Could you check a few things on this model? Use its own coordinates, in mm. A direction names the side the tool comes from. Give positions to 0.01 mm unless a question says otherwise; leave off trailing zeros. Order: outer loops, then holes, each group sorted by start corner. A loop starts at its lowest first (then second) coordinate and runs counter-clockwise, first axis right, second up. Notation, with made-up numbers: (6, 74) -> (33, 74) arc R27 ccw to (33, 100) -> close; hole circle Ø2 at (-30, 38.25). An arc over 180 degrees is marked (long way). One line per item, written item: value.
```python
from build123d import *

# Parameters (mm, degrees)
F0_W     = 20
F0_H     = 40
F0_R     = 2.75
F1_DEPTH = 4
F2_W     = 20
F2_H     = 10
F3_DEPTH = 15
F4_W     = 8.5
F4_H     = 4.5
F5_DEPTH = 30
F6_R     = 2.5
F7_DEPTH = 20
F9_DEPTH = 3


# Not quite as in the source:
# - a pattern or mirror of a feature is missing from the dataset's text; its kind, count and spacing are read off the source's solid


with BuildPart() as f1:
    # F0 (on Front) → F1 (new body)
    with BuildSketch(Plane.XZ):
        Rectangle(F0_W, F0_H)
        with Locations((0, -10)):
            Circle(F0_R, mode=Mode.SUBTRACT)
        with Locations((0, 10)):
            Circle(F0_R, mode=Mode.SUBTRACT)
    extrude(amount=F1_DEPTH)

    # F2 (on face) → F3 (join)
    with BuildSketch(Plane(origin=(0, 0, 0), x_dir=(-1, 0, 0), z_dir=(0, 1, 0))):
        with Locations((0, 20)):
            Rectangle(F2_W, F2_H)
    extrude(amount=-F3_DEPTH)

    # F4 (on face) → F5 (cut)
    with BuildSketch(Plane.XZ.offset(15)):
        with Locations((0, 20)):
            Rectangle(F4_W, F4_H)
    extrude(amount=-F5_DEPTH, mode=Mode.SUBTRACT)

    # F6 (on face) → F7 (cut)
    with BuildSketch(Plane.XY.offset(25)):
        with Locations((0, -10)):
            Circle(F6_R)
    extrude(amount=-F7_DEPTH, mode=Mode.SUBTRACT)

    # F8 (on face) → F9 (join)
    with BuildSketch(Plane(origin=(-10, 0, 0), x_dir=(0, -1, 0), z_dir=(-1, 0, 0))):
        Polygon((4, -20), (15, 15), (4, 15), align=None)
    f9 = extrude(amount=-F9_DEPTH)

    # F9_copies: F9 across plane
    add(f9.mirror(Plane(origin=(0, 0, 0), x_dir=(0, 0, 1), z_dir=(1, 0, 0))))


solid = f1.part
```
1) For P1, Ø8, axis at x = 0, y = -10, coming from the -Z side; P2, Ø9, axis at y = -10.5, z = -1.5, coming from the +X side; P3, Ø4, axis at x = 2, z = -9, coming from the -Y side, each with a flat end and sliding along its axis, tell me the tip position at first contact or that it passes through.
Answer below:
P1: stops at z = 15
P2: stops at x = 10
P3: stops at y = -4
2) Suppose I cut it at D-D, the plane x = 3.5. Write out the boundary of the cut face in (y, z).
Answer below:
outline: (-15, 15) -> (-4, 15) -> (-4, -20) -> (0, -20) -> (0, 17.75) -> (-15, 17.75) -> close; (-15, 22.25) -> (0, 22.25) -> (0, 25) -> (-15, 25) -> close
3) Suppose I cut it at C-C, the plane y = -9.25. Write out the boundary of the cut face in (x, z).
Answer below:
outline: (-10, -3.3) -> (-7, -3.3) -> (-7, 15) -> (-2.38, 15) -> (-2.38, 17.75) -> (-4.25, 17.75) -> (-4.25, 22.25) -> (-2.38, 22.25) -> (-2.38, 25) -> (-10, 25) -> close; (2.38, 15) -> (7, 15) -> (7, -3.3) -> (10, -3.3) -> (10, 25) -> (2.38, 25) -> (2.38, 22.25) -> (4.25, 22.25) -> (4.25, 17.75) -> (2.38, 17.75) -> close
4) For faces 5 (the flat face through (8.521, -9.423, -2.745)), 6 (the flat face through (4.25, -8, 20)), 7 (the flat face through (0, -7, 15)), which set-ups out of +Z, -Z, +X, -X, +Y, -Y let a thin tool reach every point of the face, with its end or its side?
Answer below:
face 5: -Z, +X, -X, -Y
face 6: +Y, -Y
face 7: -Z, -Y
5) We'd pull the mould along Z, two halves only. Please class faces 1 (the flat face through (7, -8, 2)), 2 (the flat face through (0, -6, 17.75)), 3 (the flat face through (-4.25, -8, 20)), 4 (the flat face through (-8.521, -9.423, -2.745)): +Z half, -Z half, draft (parallel to the pull), parting line (faces both ways), or undercut.
Answer below:
face 1: draft
face 2: undercut
face 3: undercut
face 4: -Z half
6) If I drill on line 1 along Z through (x, y) = (0, -0.75); line 2 along X through (y, z) = (-6.5, 3.5); line 3 along Y through (x, z) = (0, 16.15), over which ranges is the centre line in solid material (lowest first)?
Answer below:
line 1: z = -20 to -12.75, -7.25 to 7.25, 12.75 to 17.75, 22.25 to 25
line 2: x = -10 to -7, 7 to 10
line 3: y = -15 to -12.5, -7.5 to 0
7) Suppose I cut it at B-B, the plane x = 0. Write out the boundary of the cut face in (y, z).
Answer below:
outline: (-15, 15) -> (-12.5, 15) -> (-12.5, 17.75) -> (-15, 17.75) -> close; (-15, 22.25) -> (-12.5, 22.25) -> (-12.5, 25) -> (-15, 25) -> close; (-7.5, 15) -> (-4, 15) -> (-4, 12.75) -> (0, 12.75) -> (0, 17.75) -> (-7.5, 17.75) -> close; (-7.5, 22.25) -> (0, 22.25) -> (0, 25) -> (-7.5, 25) -> close; (-4, -20) -> (0, -20) -> (0, -12.75) -> (-4, -12.75) -> close; (-4, -7.25) -> (0, -7.25) -> (0, 7.25) -> (-4, 7.25) -> close
8) Suppose I cut it at A-A, the plane z = 19.5. Write out the boundary of the cut face in (x, y), then the cut area to 4 significant figures.
Answer below:
outline: (-10, -15) -> (-4.25, -15) -> (-4.25, 0) -> (-10, 0) -> close; (4.25, -15) -> (10, -15) -> (10, 0) -> (4.25, 0) -> close
area: 172.5 mm2
